The figure shows three views and two pictorial views of one solid part (mm, origin at its lowest corner). Answer the questions. A direction names the side the tool comes from. Coordinates: 2 decimals unless noted, no trailing zeros. Order: outer loops, then holes, each group sorted by start corner. A loop starts at its lowest first (then second) coordinate and runs counter-clockwise, first axis right, second up. Notation, with made-up numbers: (39.5, 7.25) - (55.5, 7.25) arc R11 ccw to (55.5, 26.25) - close; hole circle Ø8 at (26, 38). An arc over 180 degrees is marked (long way). Answer as a JSON object with one key per item and string values. Group by question number.
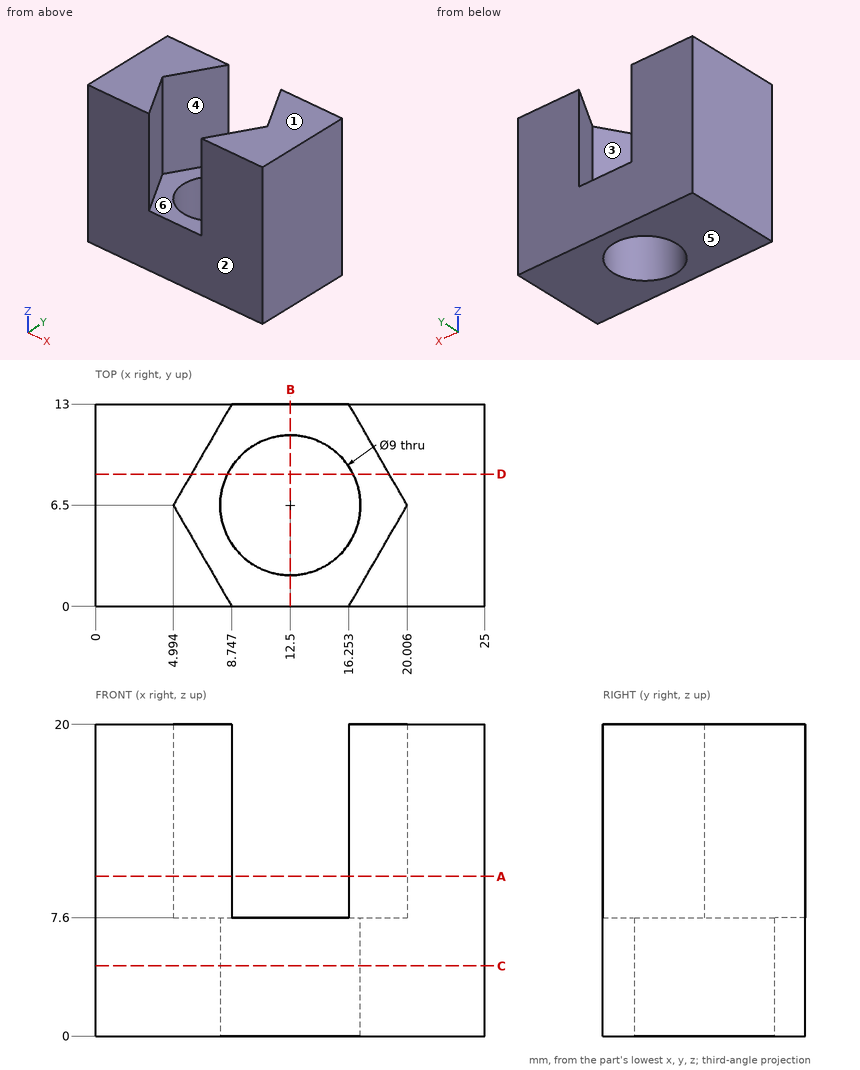
1. A cutting plane is placed at C-C on z = 4.5. Write down the section's boundary in (x, y).
2. For the marked faces 5 and 6, determine the directions among +Z, -Z, +X, -X, +Y, -Y from which every point of the face is accessible in a straight line to the end or side of a thin tool.
3. Given pin 1 (6.5 mm diameter, centred on x = 15, y = 4.5, fed in from +Z), flat-ended and moving along its own axis, determine where the tip first touches the part or whether it passes through.
4. For a pull along Y with two mould halves and no side action, classify the marked faces 1, 2, 3 and 4 as pulls with the +Y half, pulls with the -Y half, needs draft (parallel to the pull), parting line crosses it, or undercut.
5. A cutting plane is placed at A-A on z = 10.25. Write down the section's boundary in (x, y) (1 decimal), and give its area (3 significant figures).
6. A cutting plane is placed at D-D on y = 8.5. Write down the section's boundary in (x, z), and give its area (3 significant figures).
7. Straight lines are drawn through the part: L1, parallel to Y at x = 12.5, z = 3; L2, parallel to X at y = 8.25, z = 17 (1 decimal); L3, parallel to X at y = 10, z = 8.5 (1 decimal). For each, find the intervals that lie inside material, in ascending order.
8. A cutting plane is placed at B-B on x = 12.5. Write down the section's boundary in (y, z), and give its area (3 significant figures).
Derived:
{
 "1": {"outline": "(0, 0) - (25, 0) - (25, 13) - (0, 13) - close; hole circle Ø9 at (12.5, 6.5)"},
 "2": {"face 5": "-Z, +X, -X, +Y, -Y", "face 6": "+Z"},
 "3": {"pin 1": "stops at z = 7.6"},
 "4": {"face 1": "needs draft", "face 2": "pulls with the -Y half", "face 3": "undercut", "face 4": "undercut"},
 "5": {"outline": "(0, 0) - (8.7, 0) - (5, 6.5) - (8.7, 13) - (0, 13) - close; (16.3, 0) - (25, 0) - (25, 13) - (16.3, 13) - (20, 6.5) - close", "area": "179 mm2"},
 "6": {"outline": "(0, 0) - (8.47, 0) - (8.47, 7.6) - (6.15, 7.6) - (6.15, 20) - (0, 20) - close; (16.53, 0) - (25, 0) - (25, 20) - (18.85, 20) - (18.85, 7.6) - (16.53, 7.6) - close", "area": "281 mm2"},
 "7": {"L1": "y = 0 to 2, 11 to 13", "L2": "x = 0 to 6, 19 to 25", "L3": "x = 0 to 7, 18 to 25"},
 "8": {"outline": "(0, 0) - (2, 0) - (2, 7.6) - (0, 7.6) - close; (11, 0) - (13, 0) - (13, 7.6) - (11, 7.6) - close", "area": "30.4 mm2"}
}
